Autodesk Inventor part; units mm, degrees
ref_plane "YZ Plane" through (0, 0, 0) normal (1, 0, 0) x (0, 1, 0)
ref_plane "XZ Plane" through (0, 0, 0) normal (0, 1, 0) x (-1, 0, 0)
ref_plane "XY Plane" through (0, 0, 0) normal (0, 0, 1) x (1, 0, 0)
sketch "Sketch1" plane through (0, 0, 0) normal (0, 1, 0) x (-1, 0, 0)
  circle A0 centre (0, 0) radius 5
  dimension "d0" = 10
extrude "Extrusion1" add sketch "Sketch1" along normal blind 50
sketch "Sketch2" plane through (0, 0, 0) normal (1, 0, 0) x (0, 1, 0)
  line L0 (0, 5) -> (0, -5)
  line L1 (0, -5) -> (0, 0)
  line L2 (-15, 0) -> (0, 0)
  line L3 (0, -5) -> (-15, 0)
  dimension "d3" = 15
revolve "Revolution1" add sketch "Sketch2" angle 360 about axis through (0, -15, 0) along (0, 1, 0)
sketch "Sketch4" plane through (0, 0, 0) normal (1, 0, 0) x (0, 1, 0)
  line L0 (50, -5) -> (50, 5)
  arc A0 (50, -5) -> (55, 0) centre (50, 0) ccw
  line L1 (55, 0) -> (50, 0)
  line L2 (50, -5) -> (50, 0)
  point P0 (0, 0)
revolve "Revolution2" add sketch "Sketch4" angle 360 about axis through (0, 55, 0) along (0, -1, 0)
equation "\"d0\" = cylinder_r"
equation "\"d1\" = cylinder_h"
equation "\"d3\" = cone_h"
equation "\"cylinder_h\" = 50"
equation "\"cone_h\" = 15"
equation "\"cylinder_r\" = 10"
properties part number "parametrized pencile"
Input: part model. Units: mm. Frame: model coordinates. Round coordinates to 2 decimals unless told otherwise and drop trailing zeros. Loops run counter-clockwise (first coordinate to the right, second up) from the corner with the lowest first, then second, coordinate; pieces in that order, holes last.
1) Pin query (flat end, axial travel): pin 1 (1 mm diameter, centred on y = 22, z = 1.5, fed in from +X); pin 2 (1 mm diameter, centred on x = -1, z = 3.5, fed in from +Y); pin 3 (6 mm diameter, centred on x = -3.5, y = 31, fed in from +Z). Return the tip coordinate at first contact, or that it passes through.
Ans:
pin 1: stops at x = 4.9
pin 2: stops at y = 53.89
pin 3: stops at z = 4.97
2) Material intervals for line 1 (Z direction, x = 3.75, y = 33); line 2 (Y direction, x = 2, z = 1.5); line 3 (X direction, y = 14, z = -3.25), sorted ascending.
Ans:
line 1: z = -3.31 to 3.31
line 2: y = -7.5 to 54.33
line 3: x = -3.8 to 3.8
3) Section query A-A on y = 18.5. Return the cut outline in (x, z).
Ans:
outline: circle Ø10 at (0, 0)
